Geometry check sheet. Reference: the model listing, model coordinates, mm. Face numbers are marked on the shaded views. A direction names the side the tool comes from. Round coordinates to 2 decimals unless told otherwise and drop trailing zeros. Write each loop counter-clockwise with the first axis right and the second up, starting at its lowest first coordinate (ties: lowest second). Pieces come first, ordered by that corner, then holes. Notation, with made-up numbers: M 14.5,30 L 61.5,30 A23 ccw 61.5,57 Z; hole C 56,-15 d11. An arc over 180 degrees is marked long. One line per item, written item: value. Start each with the question number.
1. Section check B-B (z = 20). Count the separate pieces of the cut face and the enclosed holes in it, and give its area (3 significant figures).
2. Access from +Z, -Z, +X, -X, +Y, -Y to the whole of each face (thin tool, end or side, straight path). Record for the marked faces 5 and 6.
3. Depth check by flat-ended pin: P1, Ø7.5, axis at x = -209.65, y = 25.4, coming from the +Z side; P2, Ø5, axis at x = -193.78, y = 9.52, coming from the -Z side. Enter the tip coordinate at first touch or a pass-through.
4. Section check A-A (x = -251). Record the boundary of the cut face in (y, z).
5. Release check for a two-part mould opening along X. For the marked faces 1, 2, 3 and 4 record: pulls with the +X half, pulls with the -X half, needs draft (parallel to the pull), parting line crosses it, or undercut.
6. Scan lines: probe 1 along X at (y, z) = (9.5, 3); probe 2 along X at (y, z) = (10, 13.25); probe 3 along Z at (x, y) = (-207.5, 24.5). Record each from-to range of solid material in increasing order. Write a range as [from, to].
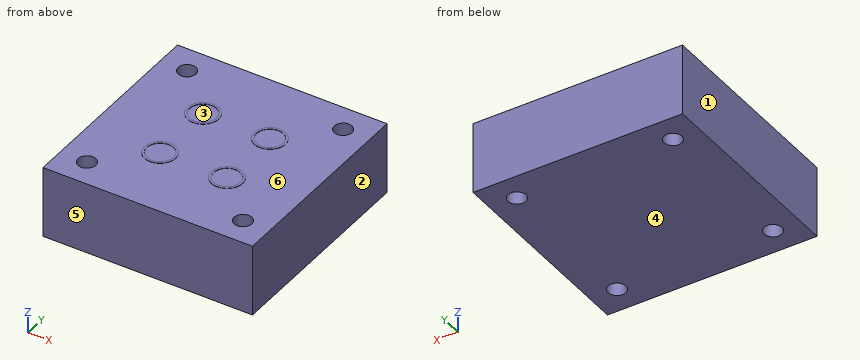
from build123d import *

# Parameters (mm, degrees)
F0_W     = 74.6125
F0_H     = 74.6125
F1_DEPTH = 25.4
F2_R     = 3.175
F3_DEPTH = 25.4
F4_R     = 5.55625
F5_DEPTH = 0.1
F6_R     = 4.7625
F7_DEPTH = 0.1


with BuildPart() as f1:
    # F0 (on Top) → F1 (new body)
    with BuildSketch(Plane.XY):
        with Locations((-221.559285, 37.30625)):
            Rectangle(F0_W, F0_H)
    extrude(amount=F1_DEPTH)

    # F2 (on Top) → F3 (cut)
    with BuildSketch(Plane.XY):
        with Locations((-249.340535, 65.0875)):
            Circle(F2_R)
        with Locations((-193.778035, 65.0875)):
            Circle(F2_R)
        with Locations((-249.340535, 9.525)):
            Circle(F2_R)
        with Locations((-193.778035, 9.525)):
            Circle(F2_R)
    extrude(amount=F3_DEPTH, mode=Mode.SUBTRACT)

    # F4 (on face) → F5 (join)
    with BuildSketch(Plane.XY.offset(25.4)):
        with Locations((-233.465535, 49.2125)):
            Circle(F4_R)
        with Locations((-209.653035, 49.2125)):
            Circle(F4_R)
        with Locations((-233.465535, 25.4)):
            Circle(F4_R)
        with Locations((-209.653035, 25.4)):
            Circle(F4_R)
    extrude(amount=F5_DEPTH)

    # F6 (on face) → F7 (cut)
    with BuildSketch(Plane.XY.offset(25.5)):
        with Locations((-233.465535, 25.4)):
            Circle(F6_R)
        with Locations((-233.465535, 49.2125)):
            Circle(F6_R)
        with Locations((-209.653035, 25.4)):
            Circle(F6_R)
        with Locations((-209.653035, 49.2125)):
            Circle(F6_R)
    extrude(amount=-F7_DEPTH, mode=Mode.SUBTRACT)


solid = f1.part
Result sheet:
1. separate pieces: 1
1. enclosed holes: 4
1. area: 5,440 mm2
2. face 5: +Z, -Z, +X, -X, -Y
2. face 6: +Z
3. P1: stops at z = 25.4
3. P2: passes through
4. outline: M 0,0 L 6.82,0 L 6.82,25.4 L 0,25.4 Z; M 12.23,0 L 62.38,0 L 62.38,25.4 L 12.23,25.4 Z; M 67.79,0 L 74.61,0 L 74.61,25.4 L 67.79,25.4 Z
5. face 1: pulls with the -X half
5. face 2: pulls with the +X half
5. face 3: undercut
5. face 4: needs draft
6. probe 1: x = [-258.87, -252.52], [-246.17, -196.95], [-190.6, -184.25]
6. probe 2: x = [-258.87, -252.48], [-246.2, -196.92], [-190.64, -184.25]
6. probe 3: z = [0, 25.4]
